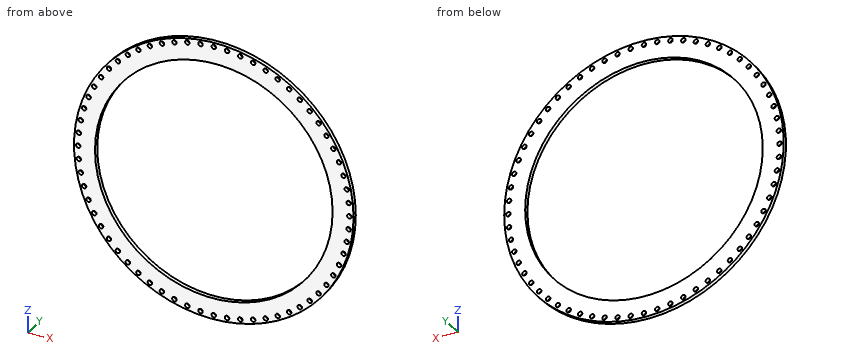
from build123d import *

# Parameters (mm, degrees)
ESQUISSE2_W                  = 100
ESQUISSE2_H                  = 3
ESQUISSE4_R                  = 85
CENTRALHOLE_DEPTH            = 4
ESQUISSE5_R                  = 1.6
FIXINGHOLE_DEPTH             = 4
R_P_TITION_CIRCULAIRE1_COUNT = 64


with BuildPart() as part:
    # Esquisse2 → MainRevolution (revolve)
    with BuildSketch(Plane.XY):
        with Locations((50, 1.5)):
            Rectangle(ESQUISSE2_W, ESQUISSE2_H)
    revolve(axis=Axis((0, 55, 0), (0, -1, 0)))

    # Esquisse4 → CentralHole (cut, through all)
    with BuildSketch(Plane(origin=(0, 3, 0), x_dir=(1, 0, 0), z_dir=(0, 1, 0))):
        Circle(ESQUISSE4_R)
    extrude(amount=-CENTRALHOLE_DEPTH, mode=Mode.SUBTRACT)

    # Esquisse5 → FixingHole (cut, through all)
    with BuildSketch(Plane(origin=(0, 3, 0), x_dir=(1, 0, 0), z_dir=(0, 1, 0))):
        with Locations((97, 0)):
            Circle(ESQUISSE5_R)
    fixinghole = extrude(amount=-FIXINGHOLE_DEPTH, mode=Mode.SUBTRACT)

    # Répétition circulaire1: FixingHole ×64 about axis
    r_p_tition_circulaire1_axis = Axis((0, 0, 0), (0, 1, 0))
    for i in range(1, R_P_TITION_CIRCULAIRE1_COUNT):
        add(fixinghole.rotate(r_p_tition_circulaire1_axis, i * 360 / R_P_TITION_CIRCULAIRE1_COUNT), mode=Mode.SUBTRACT)


solid = part.part
The listing builds one solid part. Answer for the finished solid, in the listing's coordinates (mm). Give positions to 0.01 mm unless a question says otherwise; leave off trailing zeros. One line per question, with ' | ' between items. Start each with the question number.
1. Given P1, Ø3, axis at x = 45.73, z = -85.55, coming from the -Y side; P2, Ø1, axis at x = -66.5, y = 2.5, coming from the -Z side; P3, Ø1.5, axis at x = 15.5, y = 2.5, coming from the -Z side, each flat-ended and moving along its own axis, determine where each tip first touches the part or whether it passes through.
2. Straight lines are drawn through the part: line 1 (X direction, y = 1.7, z = -92); line 2 (Z direction, x = 9.5, y = 2.2); line 3 (Z direction, x = -68.5, y = 1.45). For each, find the intervals that lie inside material, in ascending order.
3. Section A-A, the plane y = 1.9 is taken. Count the separate pieces of the cut face and the enclosed holes in it, then the cut area to 3 significant figures.
Result:
1) P1: passes through | P2: stops at z = -75.13 | P3: stops at z = -98.91
2) line 1: x = -39.19 to -29.53, -26.79 to 26.79, 29.53 to 39.19 | line 2: z = -99.55 to -98.13, -94.93 to -84.47, 84.47 to 94.93, 98.13 to 99.55 | line 3: z = -72.85 to -70.19, -66.99 to -50.33, 50.33 to 66.99, 70.19 to 72.85
3) separate pieces: 1 | enclosed holes: 65 | area: 8,200 mm2
